```python
from build123d import *

# Parameters (mm, degrees)
SKETCH_R        = 2.2
SKETCH_R_2      = 1.45
PAD_DEPTH       = 33
SKETCH037_R     = 2.2
SKETCH037_R_2   = 1.45
PAD016_DEPTH    = 4.5
SKETCH039_W     = 13.4
SKETCH039_H     = 10
PAD017_DEPTH    = 5
SKETCH045_W     = 20.9
SKETCH045_H     = 56.4
PAD018_DEPTH    = 34.6
POCKET022_DEPTH = 38.716621
SKETCH046_W     = 13.1
SKETCH046_H     = 26.8
POCKET023_DEPTH = 47.5
SKETCH047_R     = 1.5
POCKET024_DEPTH = 20.9
SKETCH041_W     = 3.4
SKETCH041_H     = 70.5
POCKET025_DEPTH = 7.3
FILLET006_R     = 0.5
FILLET007_R     = 3
FILLET008_R     = 3
FILLET009_R     = 2
FILLET010_R     = 3
FILLET011_R     = 0.5


with BuildPart() as part:
    # Sketch → Pad (new body, symmetric)
    with BuildSketch(Plane.XZ):
        with BuildLine():
            Line((-9.25, -31.677082), (9.25, -31.677082))
            ThreePointArc((9.25, -31.677082), (23.787894, -22.872168), (32.015621, -8))
            Line((-32.015621, -8), (32.015621, -8))
            ThreePointArc((-32.015621, -8), (-23.787894, -22.872168), (-9.25, -31.677082))
        make_face()
        with Locations((24.9, -12.6)):
            Circle(SKETCH_R, mode=Mode.SUBTRACT)
        with Locations((-24.9, -12.6)):
            Circle(SKETCH_R, mode=Mode.SUBTRACT)
        with Locations((0, -12.6)):
            Circle(SKETCH_R_2, mode=Mode.SUBTRACT)
        with BuildLine():
            ThreePointArc((0, -18.243174), (-6.771568, -11.057878), (-16.248592, -13.827105))
            ThreePointArc((-16.248592, -13.827105), (-21.564175, -13.876493), (-18.494342, -18.216307))
            ThreePointArc((-18.494342, -18.216307), (-11.197344, -29.424262), (0, -22.11099))
            ThreePointArc((0, -22.11099), (18.7, -20.177082), (0, -18.243174))
        make_face(mode=Mode.SUBTRACT)
    extrude(amount=PAD_DEPTH, both=True)

    # Sketch037 → Pad016 (join)
    with BuildSketch(Plane.XZ.offset(33)):
        with BuildLine():
            ThreePointArc((-32.015621, -8), (-23.787894, -22.872168), (-9.25, -31.677082))
            Line((9.25, -31.677082), (-9.25, -31.677082))
            ThreePointArc((9.25, -31.677082), (23.787894, -22.872168), (32.015621, -8))
            Line((-32.015621, -8), (32.015621, -8))
        make_face()
        with Locations((-24.9, -12.6)):
            Circle(SKETCH037_R, mode=Mode.SUBTRACT)
        with Locations((0, -12.6)):
            Circle(SKETCH037_R_2, mode=Mode.SUBTRACT)
        with Locations((24.9, -12.6)):
            Circle(SKETCH037_R, mode=Mode.SUBTRACT)
    extrude(amount=PAD016_DEPTH)

    # Sketch039 (on Face2 of Pad016) → Pad017 (join)
    with BuildSketch(Plane(origin=(0, 0, -8), x_dir=(-1, 0, 0), z_dir=(0, 0, 1))):
        with Locations((0, 32.5)):
            Rectangle(SKETCH039_W, SKETCH039_H)
    extrude(amount=PAD017_DEPTH)

    # Sketch045 (on Face2 of Pad017) → Pad018 (join)
    with BuildSketch(Plane(origin=(0, 0, -8), x_dir=(-1, 0, 0), z_dir=(0, 0, 1))):
        with Locations((-17.15, 9.3)):
            Rectangle(SKETCH045_W, SKETCH045_H)
    extrude(amount=PAD018_DEPTH)

    # Sketch040 (on Face12 of Pad018) → Pocket022 (cut, through all)
    with BuildSketch(Plane(origin=(-6.7, 0, -11), x_dir=(0, 0, -1), z_dir=(-1, 0, 0))):
        with BuildLine():
            Line((-6.224875, 30.75), (-4.775126, 30.75))
            Line((-4.775126, 30.75), (-4.262563, 31.262563))
            ThreePointArc((-4.262563, 31.262563), (-5.5, 34.25), (-6.737437, 31.262563))
            Line((-6.224875, 30.75), (-6.737437, 31.262563))
        make_face()
    extrude(amount=-POCKET022_DEPTH, mode=Mode.SUBTRACT)

    # Sketch046 (on Face9 of Pocket022) → Pocket023 (cut)
    with BuildSketch(Plane(origin=(0, 18.9, 0), x_dir=(1, 0, 0), z_dir=(0, 1, 0))):
        with Locations((17.15, -9.4)):
            Rectangle(SKETCH046_W, SKETCH046_H)
    extrude(amount=-POCKET023_DEPTH, mode=Mode.SUBTRACT)

    # Sketch047 (on Face8 of Pocket023) → Pocket024 (cut)
    with BuildSketch(Plane(origin=(27.6, 0, 0), x_dir=(0, 0, 1), z_dir=(1, 0, 0))):
        with BuildLine():
            add(Edge.make_bspline(
                [(2, -18.9), (9.3, 73.1), (16.6, -18.9)],
                knots=[-7.3, -7.3, -7.3, 7.3, 7.3, 7.3], degree=2))
            Line((16.6, -18.9), (2, -18.9))
        make_face()
        with Locations((-1.5, -14.9)):
            Circle(SKETCH047_R)
        with Locations((20.1, -14.9)):
            Circle(SKETCH047_R)
    extrude(amount=-POCKET024_DEPTH, mode=Mode.SUBTRACT)

    # Sketch041 (on Face38 of Pocket024) → Pocket025 (cut)
    with BuildSketch(Plane(origin=(0, 0, -3), x_dir=(-1, 0, 0), z_dir=(0, 0, 1))):
        with Locations((0, 2.25)):
            Rectangle(SKETCH041_W, SKETCH041_H)
    extrude(amount=-POCKET025_DEPTH, mode=Mode.SUBTRACT)

    # Fillet006
    fillet006_edges = [part.edges().sort_by_distance(p)[0] for p in [
        (-6.7, -32.5, -3),
        (1.7, -32.5, -3),
        (-1.7, -32.5, -3),
    ]]
    fillet(fillet006_edges, radius=FILLET006_R)

    # Fillet007
    fillet007_edges = [part.edges().sort_by_distance(p)[0] for p in [
        (-4.2, -27.5, -8),
        (4.2, -27.5, -8),
    ]]
    fillet(fillet007_edges, radius=FILLET007_R)

    # Fillet008
    fillet008_edges = [part.edges().sort_by_distance(p)[0] for p in [
        (27.6, -9.3, 26.6),
        (6.7, -9.3, 26.6),
    ]]
    fillet(fillet008_edges, radius=FILLET008_R)

    # Fillet009
    fillet009_edges = [part.edges().sort_by_distance(p)[0] for p in [
        (8.65, 18.9, 2),
        (25.65, 18.9, 2),
        (25.65, 18.9, 16.6),
        (8.65, 18.9, 16.6),
    ]]
    fillet(fillet009_edges, radius=FILLET009_R)

    # Fillet010
    fillet010_edges = [part.edges().sort_by_distance(p)[0] for p in [
        (17.15, 18.9, -8),
    ]]
    fillet(fillet010_edges, radius=FILLET010_R)

    # Fillet011
    fillet011_edges = [part.edges().sort_by_distance(p)[0] for p in [
        (1.7, -2.25, -10.3),
        (-1.7, -2.25, -10.3),
    ]]
    fillet(fillet011_edges, radius=FILLET011_R)


solid = part.part
```
CAD build for the part. Positions are in the model's coordinates, mm. A direction names the side the tool comes from. Give positions to 0.01 mm unless a question says otherwise; leave off trailing zeros. Loops run counter-clockwise (first coordinate to the right, second up) from the corner with the lowest first, then second, coordinate; pieces in that order, holes last. Notation, with made-up numbers: M -34.5,28 L -15.5,28 A30 cw -15.5,52 Z; hole C -34.75,68 d2. An arc over 180 degrees is marked long. Use one line per item in the form item = value.
Item 1: Flat gauge pins, fed straight in: pin 1 (9.5 mm diameter, centred on y = -9, z = 7.5, fed in from +X); pin 2 (4 mm diameter, centred on x = 15.5, y = 5.5, fed in from -Z); pin 3 (5 mm diameter, centred on y = 14.9, z = 20.1, fed in from -X); pin 4 (2.5 mm diameter, centred on x = 24.9, z = -12.6, fed in from +Y). Where does each tip first touch, or does it go through?
Determined:
pin_1 = 27.6
pin_2 = -30.11
pin_3 = 6.7
pin_4 = through
Item 2: Two-plate mould, pull along X, no slides. Class faces 1 (the face through (0, -2, -31.677)), 2 (the face through (17, -5, 22.8)), 3 (the face through (7.56, -9.69, 25.7)), 4 (the face through (17, -5, -4)): pulls with the +X half, pulls with the -X half, needs draft (parallel to the pull), parting line crosses it, or undercut.
Determined:
face_1 = needs draft
face_2 = undercut
face_3 = pulls with the -X half
face_4 = undercut
Item 3: Slice it at B-B (x = 11.5). List the corners of the cut face in (y, z), plus the area to 3 significant figures.
Determined:
outline = M -37.5,-30.93 L 33,-30.93 L 33,-29.36 L -33,-29.36 L -33,-11 L 33,-11 L 33,-8 L 21.9,-8 A3 cw 18.9,-5 L 18.9,-4 L -28.6,-4 L -28.6,22.8 L 18.9,22.8 L 18.9,26.6 L -37.5,26.6 Z; hole M -31.26,-6.74 L -30.75,-6.22 L -30.75,-4.78 L -31.26,-4.26 A1.75 ccw long Z
area = 1,080 mm2
Item 4: Slice it at C-C (y = -8). Count the separate pieces of the cut face and the enclosed holes in it, plus the area to 3 significant figures.
Determined:
separate_pieces = 2
enclosed_holes = 4
area = 839 mm2
Item 5: Drill centre lines: probe 1 along Z at (x, y) = (-4, -32); probe 2 along Z at (x, y) = (8.1, 14.9); probe 3 along X at (y, z) = (-21, 15). Where is each one in solid material? Low to high. Write a range as from..to.
Determined:
probe_1 = -31.68..-28.03, -12.32..-7.18, -3.82..-3
probe_2 = -31.68..-29.56, -10.8..-3, 0..2.32, 16.28..18.6, 21.6..26.14
probe_3 = 6.7..10.6, 23.7..27.6
Item 6: Slice it at A-A (z = -1.5). List the corners of the cut face in (x, y).
Determined:
outline = M 6.7,-37.5 L 27.6,-37.5 L 27.6,13.4 L 23.7,13.4 L 23.7,-28.6 L 10.6,-28.6 L 10.6,13.4 L 6.7,13.4 Z; M 6.7,16.4 L 10.6,16.4 L 10.6,18.9 L 6.7,18.9 Z; M 23.7,16.4 L 27.6,16.4 L 27.6,18.9 L 23.7,18.9 Z
Item 7: Which spindle directions (+Z, -Z, +X, -X, +Y, -Y) get a long thin tool onto all of the face, cutting with end or side? Do faces 5 (the face through (25.68, 14.83, 18.6)), 6 (the face through (-4.24, -26.6, -7.14)), 7 (the face through (10.6, -10, 16)), 8 (the face through (4, -33, -3)). Say none if no direction does.
Determined:
face_5 = +X, -X
face_6 = +Z, -X, +Y
face_7 = +Y
face_8 = +Z, -X, +Y, -Y
